```python
from build123d import *

# Parameters (mm, degrees)
F2_SIZE  = 0.79375
F4_DEPTH = 3.96875
F5_R     = 3.17499
F7_D     = 4.0894


# Not quite as in the source:
# - a fillet or chamfer is up to 0.001 mm smaller than in the source, because OpenCascade refuses the exact size


with BuildPart() as f1:
    # F0 (on Front) → F1 (revolve)
    with BuildSketch(Plane.XZ):
        Polygon((-6.35, -10.16), (0, -10.16), (0, 0), (-9.525, 0), (-9.525, -5.08), (-6.35, -5.08), align=None)
    revolve(axis=Axis((0, 0, -1.025330542), (0, 0, -1)))

    # F2
    f2_edges = [f1.edges().sort_by_distance(p)[0] for p in [
        (9.525, 0, 0),
        (9.525, 0, -5.08),
    ]]
    chamfer(f2_edges, length=F2_SIZE)

    # F3 (on face) → F4 (cut)
    with BuildSketch(Plane.XY):
        with BuildLine():
            Line((-4.7625, -3.175), (-1.8330871047, -3.175))
            Line((-1.8330871047, -3.175), (-0.368380657, -5.7119459855))
            ThreePointArc((-0.368380657, -5.7119459855), (3.96875, -6.8740766425), (5.130880657, -2.5369459855))
            Line((5.130880657, -2.5369459855), (3.6661742094, 0))
            Line((3.6661742094, 0), (5.130880657, 2.5369459855))
            ThreePointArc((5.130880657, 2.5369459855), (3.96875, 6.8740766425), (-0.368380657, 5.7119459855))
            Line((-0.368380657, 5.7119459855), (-1.8330871047, 3.175))
            Line((-1.8330871047, 3.175), (-4.7625, 3.175))
            ThreePointArc((-4.7625, 3.175), (-7.9375, 0), (-4.7625, -3.175))
        make_face()
    extrude(amount=-F4_DEPTH, mode=Mode.SUBTRACT)

    # F5 (radius 3.175 in the source; OpenCascade refuses exactly that, so slightly less here)
    f5_edges = [f1.edges().sort_by_distance(p)[0] for p in [
        (3.96875, 6.874077, -3.96875),
        (-1.100734, 4.443473, -3.96875),
        (-3.297794, 3.175, -3.96875),
        (-7.9375, 0, -3.96875),
        (-3.297794, -3.175, -3.96875),
        (-1.100734, -4.443473, -3.96875),
        (3.96875, -6.874077, -3.96875),
        (4.398527, -1.268473, -3.96875),
        (4.398527, 1.268473, -3.96875),
    ]]
    fillet(f5_edges, radius=F5_R)

    # F7 (through all)
    with Locations(Plane(origin=(0, 0, -10.16), x_dir=(1, 0, 0), z_dir=(0, 0, -1))):
        with Locations((0, 0)):
            Hole(F7_D / 2)


solid = f1.part
```
Model file for the job. Use its own axes, mm. A direction names the side the tool comes from. Round coordinates to 2 decimals unless told otherwise and drop trailing zeros. Loops run counter-clockwise (first coordinate to the right, second up) from the corner with the lowest first, then second, coordinate; pieces in that order, holes last. Notation, with made-up numbers: M 31.5,-22 L 78.5,-22 A16 cw 78.5,2 Z; hole C -4,54.5 d3. An arc over 180 degrees is marked long. Put each result on its own line as item: value. Start each with the question number.
Item 1: Drill centre lines: line 1 along Y through (x, z) = (0, -6); line 2 along Y through (x, z) = (-0.5, -4.5). Where is each one in solid material? Low to high.
Item 2: Mould opens along Y. For faces 1 (the face through (2, 2, -10.16)), 2 (the face through (-1.11, -4.43, -0.39)), 3 (the face through (1.38, -6.2, -7.66)) say: released by +Y, released by -Y, zero draft, split by the parting line, or undercut.
Item 3: Cut at A-A (z = -8.5). List the corners of the cut face in (x, y), then the cut area to 3 significant figures.
Item 4: Drop flat-ended pins along their axis: P1, Ø5, axis at x = 2, z = -9, coming from the -Y side; P2, Ø5, axis at y = -3.5, z = -6.5, coming from the +X side; P3, Ø1.5, axis at x = 1.5, y = -2.5, coming from the +Z side; P4, Ø5, axis at x = 2, z = -3, coming from the +Y side (3 decimals). Give the stop position or say it passes through.
Item 5: 3-axis set-ups, long thin cutter, end or side, ignore diameter. For faces 4 (the face through (4, 0, 0)), 5 (the face through (3.908, -6.908, -0.391)), 6 (the face through (6, -3, -5.08)): which of +Z, -Z, +X, -X, +Y, -Y reach the whole face in a straight line?
Answer block:
1. line 1: -6.35 to -2.04, 2.04 to 6.35
1. line 2: -9.3 to -1.98, 1.98 to 9.3
2. face 1: zero draft
2. face 2: undercut
2. face 3: split by the parting line
3. outline: C 0,0 d12.7; hole C 0,0 d4.09
3. area: 114 mm2
4. P1: y = -6.35
4. P2: x = 9.23
4. P3: z = -3.87
4. P4: y = 9.525
5. face 4: +Z, +X, -X, +Y, -Y
5. face 5: +Z
5. face 6: -Z
